```python
from build123d import *

# Parameters (mm, degrees)
SKETCH2_W           = 9.652
SKETCH2_H           = 5.334
BOSS_EXTRUDE1_DEPTH = 6.223
FILLET1_R           = 1.016
BOSS_EXTRUDE2_DEPTH = 1.5748
FILLET2_R           = 1.905


with BuildPart() as part:
    # Sketch2 → Boss-Extrude1 (new body)
    with BuildSketch(Plane(origin=(0, 0, 0), x_dir=(1, 0, 0), z_dir=(0, 1, 0))):
        Polygon((-9.652, 0), (-9.652, 5.334), (-9.652, 12.192), (-35.052, 12.192), (-35.052, -3.81), (-9.652, -3.81), align=None)
        with Locations((-4.826, 2.667)):
            Rectangle(SKETCH2_W, SKETCH2_H)
        Polygon((0, -17.416581723), (6.096, 5.334), (0, 5.334), (0, 0), align=None)
    extrude(amount=BOSS_EXTRUDE1_DEPTH)

    # Fillet1
    fillet1_edges = [part.edges().sort_by_distance(p)[0] for p in [
        (0, 3.1115, 17.416581723),
    ]]
    fillet(fillet1_edges, radius=FILLET1_R)

    # Sketch3 → Boss-Extrude2 (add)
    with BuildSketch(Plane.XZ):
        with BuildLine():
            Line((0, 9.699295544), (0, 0))
            Line((0, 0), (0, -5.334))
            Line((0, -5.334), (6.096, -5.334))
            Line((6.096, -5.334), (1.99738064, 9.962255694))
            ThreePointArc((1.99738064, 9.962255694), (0.883385389, 10.706603524), (0, 9.699295544))
        make_face()
    extrude(amount=BOSS_EXTRUDE2_DEPTH)

    # Fillet2
    fillet2_edges = [part.edges().sort_by_distance(p)[0] for p in [
        (6.096, 2.3241, -5.334),
    ]]
    fillet(fillet2_edges, radius=FILLET2_R)


solid = part.part
```
Check sheet for the modelled part. Datum: model origin and axes. Units: mm. A direction names the side the tool comes from. Round coordinates to 2 decimals unless told otherwise and drop trailing zeros. Order: outer loops, then holes, each group sorted by start corner. A loop starts at its lowest first (then second) coordinate and runs counter-clockwise, first axis right, second up.
1) Scan lines: line 1 (Y direction, x = -29.5, z = -6.75); line 2 (X direction, y = 0.75, z = -6.5); line 3 (Z direction, x = -13.5, y = 5). Record each from-to range of solid material in increasing order.
2) Section check D-D (x = -5.5). Record the boundary of the cut face in (y, z), and give its area (3 significant figures).
3) Mould release check, pull along X, two halves, no side actions. Record for faces 6 (the flat face through (-35.052, 3, -4)), 7 (the flat face through (-22, 0, -4)), 8 (the flat face through (-9.652, 3, 2)), 9 (the flat face through (0, 2, 4)): +X half, -X half, draft (parallel to the pull), parting line (faces both ways), or undercut.
4) Tool access check on faces 1 (the flat face through (-20, 6.223, -3)), 2 (the flat face through (-22, 3, -12.192)), 3 (the flat face through (-5, 3, 0)), 4 (the flat face through (-3, 3, -5.334)), 5 (the flat face through (-23, 3, 3.81)). Record the directions out of +Z, -Z, +X, -X, +Y, -Y that give a thin tool (end or side, any length) a straight path to the whole face; none if there is none.
5) Section check A-A (y = 5). Record the boundary of the cut face in (x, z) (3 decimals), and give its area (3 significant figures).
6) Section check C-C (z = -1.75). Record the boundary of the cut face in (x, y), and give its area (3 significant figures).
7) Go/stop test with flat-tipped pins: pin 1 Ø3 at (y, z) = (4.5, -9.5) entering from +X; pin 2 Ø2.5 at (x, y) = (-1, 3) entering from -Z; pin 3 Ø1.1 at (y, z) = (2.5, 1.5) entering from +X; pin 4 Ø2.5 at (y, z) = (1, 4) entering from -X. Record where each tip stops, or that it passes through.
8) Section check B-B (z = 1.75). Record the boundary of the cut face in (x, y).
Result:
1. line 1: y = 0 to 6.22
1. line 2: x = -35.05 to -9.65
1. line 3: z = -12.19 to 3.81
2. outline: (0, -5.33) - (6.22, -5.33) - (6.22, 0) - (0, 0) - close
2. area: 33.2 mm2
3. face 6: -X half
3. face 7: draft
3. face 8: undercut
3. face 9: undercut
4. face 1: +Z, -Z, +X, -X, +Y
4. face 2: -Z, +X, -X, +Y, -Y
4. face 3: +Z, +Y, -Y
4. face 4: -Z, +X, +Y, -Y
4. face 5: +Z, -X, +Y, -Y
5. outline: (-35.052, -12.192) - (-9.652, -12.192) - (-9.652, -5.334) - (3.613, -5.334) arc R1.905 ccw to (5.453, -2.936) - (1.997, 9.962) arc R1.016 ccw to (0, 9.699) - (0, 0) - (-9.652, 0) - (-9.652, 3.81) - (-35.052, 3.81) - close
5. area: 520 mm2
6. outline: (-35.05, 0) - (0, 0) - (0, -1.57) - (5.14, -1.57) - (5.14, 6.22) - (-35.05, 6.22) - close
6. area: 258 mm2
7. pin 1: stops at x = -9.65
7. pin 2: stops at z = -5.33
7. pin 3: stops at x = 4.41
7. pin 4: stops at x = -35.05
8. outline: (-35.05, 0) - (-9.65, 0) - (-9.65, 6.22) - (-35.05, 6.22) - close; (0, -1.57) - (4.2, -1.57) - (4.2, 6.22) - (0, 6.22) - close
